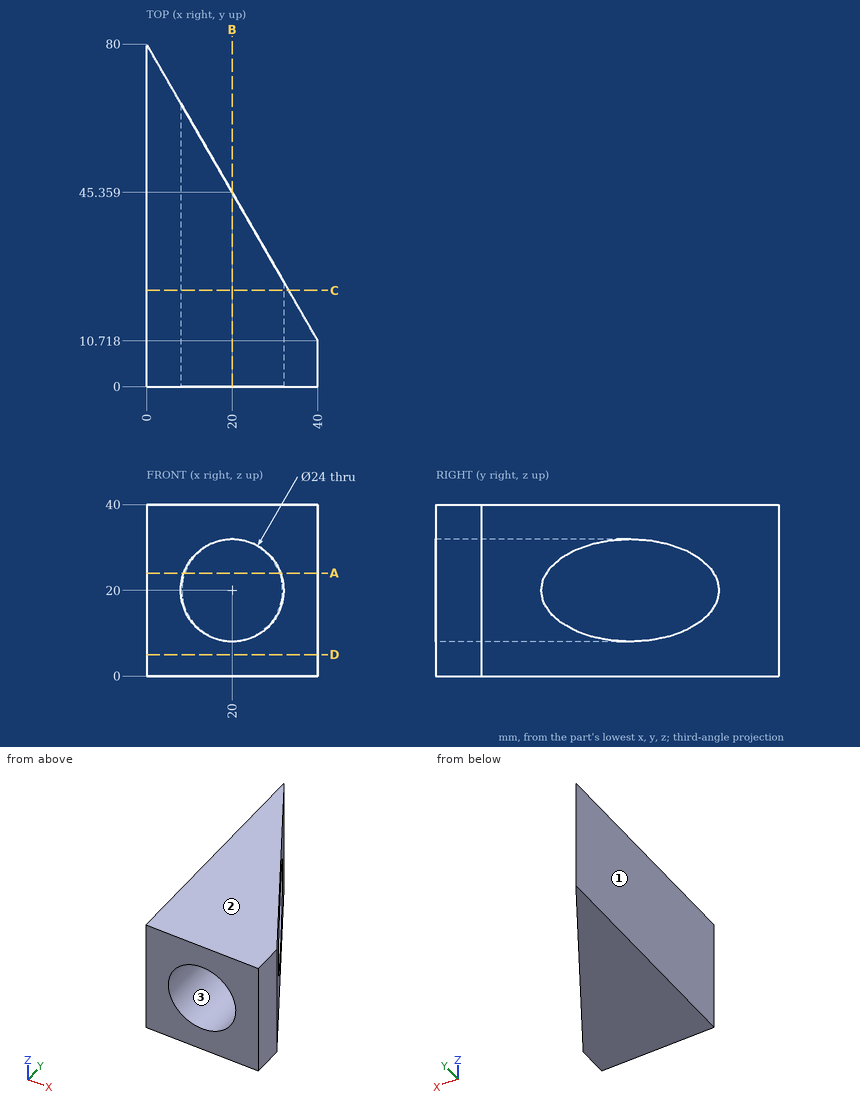
Print and shaded views of the part. All mm, measured from the part's lowest x, y and z. Coordinates: 2 decimals unless noted, no trailing zeros. Order: outer loops, then holes, each group sorted by start corner. A loop starts at its lowest first (then second) coordinate and runs counter-clockwise, first axis right, second up. Notation, with made-up numbers: M 89,11 L 103,11 A17 ccw 103,38 Z; hole C -37,-26 d11. An arc over 180 degrees is marked long. Answer as CSV lines item,"result".
1) Cut at D-D (z = 5). List the corners of the cut face in (x, y).
Verdict:
outline,"M 0,0 L 40,0 L 40,10.72 L 0,80 Z"
2) Drill centre lines: L1, parallel to Z at x = 20, y = 14; L2, parallel to Z at x = 9, y = 30; L3, parallel to X at y = 27, z = 20. Where is each one in solid material? Low to high. Write a range as from..to.
Verdict:
L1,"0..8, 32..40"
L2,"0..15.2, 24.8..40"
L3,"0..8"
3) Cut at C-C (y = 22.5). List the corners of the cut face in (x, z).
Verdict:
outline,"M 0,0 L 33.2,0 L 33.2,40 L 0,40 Z; hole C 20,20 d24"
4) Cut at A-A (z = 24). List the corners of the cut face in (x, y), then the cut area to 3 significant figures.
Verdict:
outline,"M 0,0 L 8.69,0 L 8.69,64.95 L 0,80 Z; M 31.31,0 L 40,0 L 40,10.72 L 31.31,25.76 Z"
area,"788 mm2"
5) Flat gauge pins, fed straight in: P1, Ø2, axis at y = 28.5, z = 18.5, coming from the +X side; P2, Ø10, axis at y = 52, z = 32.5, coming from the +X side; P3, Ø3, axis at x = 4.5, z = 5.5, coming from the +Y side. Where does each tip first touch, or does it go through?
Verdict:
P1,"x = 8.26"
P2,"x = 19.05"
P3,"y = 74.8"
6) Mould opens along Z. For the marked faces 1, 2 and 3 say: released by +Z, released by -Z, zero draft, split by the parting line, or undercut.
Verdict:
face 1,"zero draft"
face 2,"released by +Z"
face 3,"undercut"
7) Cut at B-B (x = 20). List the corners of the cut face in (y, z).
Verdict:
outline,"M 0,0 L 45.36,0 L 45.36,8 L 0,8 Z; M 0,32 L 45.36,32 L 45.36,40 L 0,40 Z"
